Read the model definition and answer for the solid it produces. Units are mm, in the model's axes. A direction names the side the tool comes from. Coordinates: 2 decimals unless noted, no trailing zeros. Order: outer loops, then holes, each group sorted by start corner. A loop starts at its lowest first (then second) coordinate and runs counter-clockwise, first axis right, second up.
```python
from build123d import *

# Parameters (mm, degrees)
PAD_DEPTH    = 7
SKETCH001_R  = 1.7
POCKET_DEPTH = 5
FILLET_R     = 1


with BuildPart() as part:
    # Sketch → Pad (new body)
    with BuildSketch(Plane.XY):
        Polygon((-4, 3), (-4, 16.494625), (6.578848, 27.073473), (8.700169, 24.952153), (1.629101, 17.881085), (5.235345, 14.274841), (12.306413, 21.345908), (14.427734, 19.224588), (5.101573, 9.898427), (0, 15), (0, 0), (-11, 0), (-11, 3), align=None)
    extrude(amount=PAD_DEPTH)

    # Sketch001 → Pocket (cut)
    with BuildSketch(Plane(origin=(0, 3, 0), x_dir=(-1, 0, 0), z_dir=(0, 1, 0))):
        with Locations((7.500211, 3.503477)):
            Circle(SKETCH001_R)
    extrude(amount=-POCKET_DEPTH, mode=Mode.SUBTRACT)

    # Fillet
    fillet_edges = [part.edges().sort_by_distance(p)[0] for p in [
        (8.700169, 24.952153, 3.5),
        (12.306413, 21.345908, 3.5),
        (7.639509, 26.012813, 7),
        (1.289424, 21.784049, 7),
        (6.578848, 27.073473, 3.5),
        (7.639509, 26.012813, 0),
        (1.289424, 21.784049, 0),
        (13.367073, 20.285248, 7),
        (13.367073, 20.285248, 0),
        (14.427734, 19.224588, 3.5),
        (9.764653, 14.561508, 7),
        (9.764653, 14.561508, 0),
        (-4, 16.494625, 3.5),
    ]]
    fillet(fillet_edges, radius=FILLET_R)


solid = part.part
```
1) Straight lines are drawn through the part: line 1 (X direction, y = 14.75, z = 6.5); line 2 (X direction, y = 6.5, z = 1.25); line 3 (X direction, y = 15.75, z = 3.75). For each, find the intervals that lie inside material, in ascending order.
A:
line 1: x = -4 to 0, 0.25 to 4.76, 5.71 to 9.76
line 2: x = -4 to 0
line 3: x = -4 to 3.76, 6.71 to 10.95
2) Determine the mould class of faces 4 (the cylindrical face through (6.57, 26.66, 3.54)), 5 (the flat face through (9.471, 14.268, 3.465)), 6 (the flat face through (4.86, 21.11, 3.45)) for opening direction Y: pulls with the +Y half, pulls with the -Y half, needs draft (parallel to the pull), parting line crosses it, or undercut.
A:
face 4: pulls with the +Y half
face 5: pulls with the -Y half
face 6: undercut
3) Flat-ended cylindrical pins translate along their axes: pin 1 Ø4 at (y, z) = (8.5, 3.5) entering from -X; pin 2 Ø2 at (y, z) = (9, 2.5) entering from +X; pin 3 Ø1.5 at (y, z) = (3.5, 1) entering from -X; pin 4 Ø1.5 at (y, z) = (5, 4) entering from +X. Find the tip coordinate at first contact, or state that the pin passes through.
A:
pin 1: stops at x = -4
pin 2: stops at x = 5.2
pin 3: stops at x = -11
pin 4: stops at x = 0
4) A cutting plane is placed at C-C, the plane y = 2.5. Determine the outline of the cut face in (x, z), and give its area (3 significant figures).
A:
outline: (-11, 0) - (0, 0) - (0, 7) - (-11, 7) - close; hole circle Ø3.4 at (-7.5, 3.5)
area: 67.9 mm2
5) A cutting plane is placed at A-A, the plane z = 3. Determine the outline of the cut face in (x, y), and give its area (3 significant figures).
A:
outline: (-11, 0) - (-9.12, 0) - (-9.12, 3) - (-11, 3) - close; (-5.88, 0) - (0, 0) - (0, 15) - (5.1, 9.9) - (13.72, 18.52) arc R1 ccw to (13.72, 19.93) - (13.01, 20.64) arc R1 ccw to (11.6, 20.64) - (5.24, 14.27) - (1.63, 17.88) - (7.99, 24.25) arc R1 ccw to (7.99, 25.66) - (7.29, 26.37) arc R1 ccw to (5.87, 26.37) - (-3.71, 16.79) arc R1 ccw to (-4, 16.08) - (-4, 3) - (-5.88, 3) - close
area: 172 mm2
6) A cutting plane is placed at B-B, the plane x = -7.75. Determine the outline of the cut face in (y, z), and give its area (3 significant figures).
A:
outline: (0, 0) - (3, 0) - (3, 1.82) - (0, 1.82) - close; (0, 5.19) - (3, 5.19) - (3, 7) - (0, 7) - close
area: 10.9 mm2
7) Which of the six approach directions +Z, -Z, +X, -X, +Y, -Y give full straight-line access (tool end or side, diameter ignored) to faces 1 (the flat face through (3.41, 16.1, 3.45)), 2 (the flat face through (3, 12, 3)), 3 (the cylindrical face through (9.138, 14.36, 0.285))?
A:
face 1: +Z, -Z
face 2: +Z, -Z, -Y
face 3: -Z, +X, -Y
